The listing builds one solid part. Answer for the finished solid, in the listing's coordinates (mm). A direction names the side the tool comes from. Give positions to 0.01 mm unless a question says otherwise; leave off trailing zeros. Order: outer loops, then holes, each group sorted by start corner. A loop starts at its lowest first (then second) coordinate and runs counter-clockwise, first axis right, second up. Notation, with made-up numbers: (-29.75, 86.25) - (21.25, 86.25) arc R19 cw to (21.25, 115.25) - close; hole circle Ø3 at (62.25, -27.75). An arc over 180 degrees is marked (long way). Use a Markdown table: item, result. Add a question column.
1) Straight lines are drawn through the part: line 1 (X direction, y = 2.25, z = 19); line 2 (X direction, y = 1.5, z = -18); line 3 (X direction, y = -6.75, z = 4.5). For each, find the intervals that lie inside material, in ascending order.
2) Find section C-C, the plane z = -21. Determine the outline of the cut face in (x, y), plus the area to 3 significant figures.
3) Flat-ended cylindrical pins translate along their axes: pin 1 (4.5 mm diameter, centred on x = 43, z = 19.32, fed in from +Y); pin 2 (1.5 mm diameter, centred on x = -0.5, z = -10.5, fed in from +Y). Find the tip coordinate at first contact, or state that the pin passes through.
4) The mould has two halves that part along X. Classify faces 1 (the face through (-38.505, 0.112, -17.662)), 2 (the face through (49.354, 0, 0)), 3 (the face through (-41.17, 0.11, -23.82)): released by +X, released by -X, zero draft, split by the parting line, or undercut.
5) Find section A-A, the plane x = 0. Determine the outline of the cut face in (y, z), plus the area to 3 significant figures.
6) Find section B-B, the plane y = 1. Determine the outline of the cut face in (x, z).
7) For faces 4 (the face through (0.91, -3.94, 17.32)), 5 (the face through (11, 2.032, 0)), 6 (the face through (-42.983, 0, 0)), determine the directions among +Z, -Z, +X, -X, +Y, -Y from which every point of the face is accessible in a straight line to the end or side of a thin tool.
8) Find section D-D, the plane x = -35.5. Determine the outline of the cut face in (y, z), plus the area to 3 significant figures.
from build123d import *

# Parameters (mm, degrees)
F0_R     = 17.4971354571
F0_R_2   = 11.8450866669
F0_R_3   = 5.7656301988
F1_DEPTH = 2.032
F0_R_4   = 2.5396522034
F2_DEPTH = 8
F3_DEPTH = 8


# Not quite as in the source:
# - a feature names something its author has since deleted; it is built from what else it names


with BuildPart() as f1:
    # F0 (on Front) → F1 (new body)
    with BuildSketch(Plane.XZ):
        with Locations((3.1854841864, -0.0279111721)):
            Circle(F0_R)
        with Locations((3.1854841864, -0.0279111721)):
            Circle(F0_R_2, mode=Mode.SUBTRACT)
        with Locations((3.1854841864, -0.0279111721)):
            Circle(F0_R_2)
        with Locations((3.1854841864, -0.0279111721)):
            Circle(F0_R_3, mode=Mode.SUBTRACT)
    extrude(amount=-F1_DEPTH)

    # F0 (on Front) → F2 (join)
    with BuildSketch(Plane.XZ):
        with BuildLine():
            ThreePointArc((-42.9830769071, -19.3787951119), (-41.1232049677, -23.8689231724), (-36.6330769071, -25.7287951119))
            Line((-36.6330769071, -25.7287951119), (43.0040508678, -25.7287951119))
            ThreePointArc((43.0040508678, -25.7287951119), (47.4941789284, -23.8689231724), (49.3540508678, -19.3787951119))
            Line((49.3540508678, -19.3787951119), (49.3540508678, 19.3229727678))
            ThreePointArc((49.3540508678, 19.3229727678), (47.4941772917, 23.8131047796), (43.0040452799, 25.6729783557))
            Line((43.0040452799, 25.6729783557), (-36.6330769071, 25.6729783557))
            ThreePointArc((-36.6330769071, 25.6729783557), (-41.1232049677, 23.8131064163), (-42.9830769071, 19.3229783557))
            Line((-42.9830769071, 19.3229783557), (-42.9830769071, -19.3787951119))
        make_face()
        with Locations((-36.6330769071, -19.3787951119)):
            Circle(F0_R_4, mode=Mode.SUBTRACT)
        with Locations((3.1854841864, -0.0279111721)):
            Circle(F0_R, mode=Mode.SUBTRACT)
        with Locations((43.0040452799, -19.3787951119)):
            Circle(F0_R_4, mode=Mode.SUBTRACT)
        with Locations((-36.6330769071, 19.3229727678)):
            Circle(F0_R_4, mode=Mode.SUBTRACT)
        with Locations((43.0040452799, 19.3229727678)):
            Circle(F0_R_4, mode=Mode.SUBTRACT)
    extrude(amount=-F2_DEPTH)

    # F0 (on Front) → F3 (join)
    with BuildSketch(Plane.XZ):
        with BuildLine():
            ThreePointArc((-42.9830769071, -19.3787951119), (-41.1232049677, -23.8689231724), (-36.6330769071, -25.7287951119))
            Line((-36.6330769071, -25.7287951119), (43.0040508678, -25.7287951119))
            ThreePointArc((43.0040508678, -25.7287951119), (47.4941789284, -23.8689231724), (49.3540508678, -19.3787951119))
            Line((49.3540508678, -19.3787951119), (49.3540508678, 19.3229727678))
            ThreePointArc((49.3540508678, 19.3229727678), (47.4941772917, 23.8131047796), (43.0040452799, 25.6729783557))
            Line((43.0040452799, 25.6729783557), (-36.6330769071, 25.6729783557))
            ThreePointArc((-36.6330769071, 25.6729783557), (-41.1232049677, 23.8131064163), (-42.9830769071, 19.3229783557))
            Line((-42.9830769071, 19.3229783557), (-42.9830769071, -19.3787951119))
        make_face()
        with Locations((-36.6330769071, -19.3787951119)):
            Circle(F0_R_4, mode=Mode.SUBTRACT)
        with Locations((3.1854841864, -0.0279111721)):
            Circle(F0_R, mode=Mode.SUBTRACT)
        with Locations((43.0040452799, -19.3787951119)):
            Circle(F0_R_4, mode=Mode.SUBTRACT)
        with Locations((-36.6330769071, 19.3229727678)):
            Circle(F0_R_4, mode=Mode.SUBTRACT)
        with Locations((43.0040452799, 19.3229727678)):
            Circle(F0_R_4, mode=Mode.SUBTRACT)
    extrude(amount=F3_DEPTH)


solid = f1.part
The answers:
| question | item | result |
|---|---|---|
| 1 | line 1 | -42.98 to -39.15, -34.11 to 40.49, 45.52 to 49.35 |
| 1 | line 2 | -42.98 to -38.77, -34.5 to 40.87, 45.14 to 49.35 |
| 1 | line 3 | -42.98 to -13.72, 20.09 to 49.35 |
| 2 | outline | (-42.77, -8) - (-38.59, -8) - (-38.59, 8) - (-42.77, 8) - close; (-34.68, -8) - (41.05, -8) - (41.05, 8) - (-34.68, 8) - close; (44.96, -8) - (49.14, -8) - (49.14, 8) - (44.96, 8) - close |
| 2 | area | 1,350 mm2 |
| 3 | pin 1 | through |
| 3 | pin 2 | y = 2.03 |
| 4 | face 1 | undercut |
| 4 | face 2 | released by +X |
| 4 | face 3 | released by -X |
| 5 | outline | (-8, -25.73) - (8, -25.73) - (8, -17.23) - (2.03, -17.23) - (2.03, -4.83) - (0, -4.83) - (0, -17.23) - (-8, -17.23) - close; (-8, 17.18) - (0, 17.18) - (0, 4.78) - (2.03, 4.78) - (2.03, 17.18) - (8, 17.18) - (8, 25.67) - (-8, 25.67) - close |
| 5 | area | 322 mm2 |
| 6 | outline | (-42.98, -19.38) arc R6.35 ccw to (-36.63, -25.73) - (43, -25.73) arc R6.35 ccw to (49.35, -19.38) - (49.35, 19.32) arc R6.35 ccw to (43, 25.67) - (-36.63, 25.67) arc R6.35 ccw to (-42.98, 19.32) - close; hole circle Ø5.08 at (-36.63, -19.38); hole circle Ø5.08 at (-36.63, 19.32); hole circle Ø11.53 at (3.19, -0.03); hole circle Ø5.08 at (43, -19.38); hole circle Ø5.08 at (43, 19.32) |
| 7 | face 4 | -Y |
| 7 | face 5 | +Y |
| 7 | face 6 | +Z, -Z, -X, +Y, -Y |
| 8 | outline | (-8, -25.73) - (8, -25.73) - (8, -21.65) - (-8, -21.65) - close; (-8, -17.11) - (8, -17.11) - (8, 17.05) - (-8, 17.05) - close; (-8, 21.6) - (8, 21.6) - (8, 25.67) - (-8, 25.67) - close |
| 8 | area | 677 mm2 |
